```python
from build123d import *

# Parameters (mm, degrees)
SALIENTE_EXTRUIR1_DEPTH = 2.5


with BuildPart() as part:
    # Croquis1 → Saliente-Extruir1 (new body)
    with BuildSketch(Plane(origin=(0, 0, 0), x_dir=(1, 0, 0), z_dir=(0, 1, 0))):
        with BuildLine():
            Line((-2.5, 33.5), (12.3, 33.5))
            ThreePointArc((12.3, 33.5), (13.007106781, 33.207106781), (13.3, 32.5))
            Line((13.3, 32.5), (13.3, 28.5))
            Line((13.3, 28.5), (10.8, 28.5))
            Line((10.8, 28.5), (10.8, 1))
            ThreePointArc((10.8, 1), (10.507106781, 0.292893219), (9.8, 0))
            Line((9.8, 0), (0, 0))
            ThreePointArc((0, 0), (-0.707106781, 0.292893219), (-1, 1))
            Line((-1, 1), (-1, 28.5))
            Line((-1, 28.5), (-3.5, 28.5))
            Line((-3.5, 28.5), (-3.5, 32.5))
            ThreePointArc((-3.5, 32.5), (-3.207106781, 33.207106781), (-2.5, 33.5))
        make_face()
        with BuildLine():
            ThreePointArc((6.9, 23), (4.9, 25), (2.9, 23))
            Line((2.9, 23), (2.9, 19))
            ThreePointArc((2.9, 19), (4.9, 17), (6.9, 19))
            Line((6.9, 19), (6.9, 23))
        make_face(mode=Mode.SUBTRACT)
        with BuildLine():
            ThreePointArc((6.9, 5), (4.9, 7), (2.9, 5))
            Line((2.9, 5), (2.9, 4))
            ThreePointArc((2.9, 4), (4.9, 2), (6.9, 4))
            Line((6.9, 4), (6.9, 5))
        make_face(mode=Mode.SUBTRACT)
    extrude(amount=SALIENTE_EXTRUIR1_DEPTH)


solid = part.part
```
Work out the finished part from the listing and answer in its coordinate system (mm). A direction names the side the tool comes from. Round coordinates to 2 decimals unless told otherwise and drop trailing zeros. Write each loop counter-clockwise with the first axis right and the second up, starting at its lowest first coordinate (ties: lowest second). Pieces come first, ordered by that corner, then holes.
1) A cutting plane is placed at D-D on z = -3.5. Determine the outline of the cut face in (x, y), and give its area (3 significant figures).
2) A cutting plane is placed at C-C on y = 1.6. Determine the outline of the cut face in (x, z), and give its area (3 significant figures).
3) A cutting plane is placed at A-A on z = -22.5. Determine the outline of the cut face in (x, y).
4) A cutting plane is placed at B-B on x = 4.9. Determine the outline of the cut face in (y, z), and give its area (4 significant figures).
5) Flat-ended cylindrical pins translate along their axes: P1, Ø1.2, axis at y = 1.5, z = -21, coming from the -X side; P2, Ø1.2, axis at y = 1, z = -17, coming from the +X side. Find the tip coordinate at first contact, or state that the pin passes through.
6) Consider probe 1 along X at (y, z) = (0.2, -4); probe 2 along Z at (x, y) = (3.25, 0.65); probe 3 along Z at (x, y) = (4.5, 0.3). Determine where each line is inside the solid, lowest interval first.
7) Determine the mould class of faces 4 (the face through (7, 0, -17)), 5 (the face through (4.9, 1.2, -7)), 6 (the face through (-1, 1, -15)) for opening direction X: pulls with the +X half, pulls with the -X half, needs draft (parallel to the pull), parting line crosses it, or undercut.
8) Which of the six approach directions +Z, -Z, +X, -X, +Y, -Y give full straight-line access (tool end or side, diameter ignored) to faces 1 (the face through (-2, 1, -28.5)), 2 (the face through (4.9, 1.2, -2)), 3 (the face through (12, 1, -28.5))?
Entries:
1. outline: (-1, 0) - (2.96, 0) - (2.96, 2.5) - (-1, 2.5) - close; (6.84, 0) - (10.8, 0) - (10.8, 2.5) - (6.84, 2.5) - close
1. area: 19.8 mm2
2. outline: (-3.5, -32.5) arc R1 ccw to (-2.5, -33.5) - (12.3, -33.5) arc R1 ccw to (13.3, -32.5) - (13.3, -28.5) - (10.8, -28.5) - (10.8, -1) arc R1 ccw to (9.8, 0) - (0, 0) arc R1 ccw to (-1, -1) - (-1, -28.5) - (-3.5, -28.5) - close; hole (2.9, -23) arc R2 ccw to (6.9, -23) - (6.9, -19) arc R2 ccw to (2.9, -19) - close; hole (2.9, -5) arc R2 ccw to (6.9, -5) - (6.9, -4) arc R2 ccw to (2.9, -4) - close
2. area: 374 mm2
3. outline: (-1, 0) - (2.9, 0) - (2.9, 2.5) - (-1, 2.5) - close; (6.9, 0) - (10.8, 0) - (10.8, 2.5) - (6.9, 2.5) - close
4. outline: (0, -33.5) - (2.5, -33.5) - (2.5, -25) - (0, -25) - close; (0, -17) - (2.5, -17) - (2.5, -7) - (0, -7) - close; (0, -2) - (2.5, -2) - (2.5, 0) - (0, 0) - close
4. area: 51.25 mm2
5. P1: stops at x = -1
5. P2: stops at x = 10.8
6. probe 1: x = -1 to 2.9, 6.9 to 10.8
6. probe 2: z = -33.5 to -24.13, -17.87 to -6.13, -2.87 to 0
6. probe 3: z = -33.5 to -24.96, -17.04 to -6.96, -2.04 to 0
7. face 4: needs draft
7. face 5: undercut
7. face 6: pulls with the -X half
8. face 1: +Z, -X, +Y, -Y
8. face 2: +Y, -Y
8. face 3: +Z, +X, +Y, -Y
